```python
from build123d import *

# Parameters (mm, degrees)
SKETCH1_R           = 6.3627
BOSS_EXTRUDE1_DEPTH = 3.048
FILLET1_R           = 1.27


with BuildPart() as part:
    # Sketch1 → Boss-Extrude1 (new body, symmetric)
    with BuildSketch(Plane.XY):
        with BuildLine():
            ThreePointArc((-44.45, -20.32), (-30.440021806, -27.674009584), (-19.05, -38.657103373))
            Line((-19.05, -38.657103373), (-19.05, 38.657103373))
            ThreePointArc((-19.05, 38.657103373), (-30.440021806, 27.674009584), (-44.45, 20.32))
            ThreePointArc((-44.45, 20.32), (-30.081590206, 14.368409794), (-24.13, 0))
            ThreePointArc((-24.13, 0), (-30.081590206, -14.368409794), (-44.45, -20.32))
        make_face()
        with BuildLine():
            ThreePointArc((-19.05, -38.657103373), (-17.322621511, -40.998313496), (-15.719319348, -43.426177466))
            ThreePointArc((-15.719319348, -43.426177466), (1.415517775, -24.650338319), (7.62, 0))
            ThreePointArc((7.62, 0), (1.415517775, 24.650338319), (-15.719319348, 43.426177466))
            ThreePointArc((-15.719319348, 43.426177466), (-17.322621511, 40.998313496), (-19.05, 38.657103373))
            Line((-19.05, 38.657103373), (-19.05, -38.657103373))
        make_face()
        with BuildLine():
            ThreePointArc((-15.719319348, -43.426177466), (-9.406121761, -57.631125381), (-7.246114065, -73.025))
            Line((-7.246114065, -73.025), (19.05, -73.025))
            Line((19.05, -73.025), (19.05, 73.025))
            Line((19.05, 73.025), (-7.246114065, 73.025))
            ThreePointArc((-7.246114065, 73.025), (-9.406121761, 57.631125381), (-15.719319348, 43.426177466))
            ThreePointArc((-15.719319348, 43.426177466), (1.415517775, 24.650338319), (7.62, 0))
            ThreePointArc((7.62, 0), (1.415517775, -24.650338319), (-15.719319348, -43.426177466))
        make_face()
        with Locations((6.35, -60.325)):
            Circle(SKETCH1_R, mode=Mode.SUBTRACT)
        with Locations((6.35, 60.325)):
            Circle(SKETCH1_R, mode=Mode.SUBTRACT)
    extrude(amount=BOSS_EXTRUDE1_DEPTH, both=True)

    # Fillet1
    fillet1_edges = [part.edges().sort_by_distance(p)[0] for p in [
        (-44.45, -20.32, 0),
        (-44.45, 20.32, 0),
    ]]
    fillet(fillet1_edges, radius=FILLET1_R)


solid = part.part
```
Could you check a few things on this model? Use its own coordinates, in mm. Coordinates: 2 decimals unless noted, no trailing zeros. Write each loop counter-clockwise with the first axis right and the second up, starting at its lowest first coordinate (ties: lowest second). Pieces come first, ordered by that corner, then holes. Notation, with made-up numbers: (-30.75, -29.75) -> (-6.75, -29.75) arc R20 cw to (-6.75, -16.75) -> close; hole circle Ø5 at (48.25, 89.5). An arc over 180 degrees is marked (long way). Return JSON: item names as keys, results as strings.
(1) Imagine slicing it at B-B, the plane x = -33.5. Please give me the cut outline in (y, z), then the cut area to 3 significant figures.
Numbers:
{"outline": "(-25.61, -3.05) -> (-17.12, -3.05) -> (-17.12, 3.05) -> (-25.61, 3.05) -> close; (17.12, -3.05) -> (25.61, -3.05) -> (25.61, 3.05) -> (17.12, 3.05) -> close", "area": "104 mm2"}
(2) I need wall thicknesses on L1, parallel to Y at x = 6.35, z = -1.7 (3 decimals); L2, parallel to Y at x = 3, z = -0.5 (3 decimals); L3, parallel to X at y = 64, z = 0. Which ranges of each line are inside material? Lowest first, please.
Numbers:
{"L1": "y = -73.025 to -66.688, -53.962 to 53.962, 66.688 to 73.025", "L2": "y = -73.025 to -65.734, -54.916 to 54.916, 65.734 to 73.025", "L3": "x = -7.98 to 1.16, 11.54 to 19.05"}
(3) Imagine slicing it at A-A, the plane x = 6.35. Please give me the cut outline in (y, z) (3 decimals).
Numbers:
{"outline": "(-73.025, -3.048) -> (-66.688, -3.048) -> (-66.688, 3.048) -> (-73.025, 3.048) -> close; (-53.962, -3.048) -> (53.962, -3.048) -> (53.962, 3.048) -> (-53.962, 3.048) -> close; (66.688, -3.048) -> (73.025, -3.048) -> (73.025, 3.048) -> (66.688, 3.048) -> close"}
(4) I'm going to push flat-ended pins straight in: pin 1 (2 mm diameter, centred on x = -32, z = -0.5, fed in from +Y); pin 2 (1 mm diameter, centred on x = -32, z = -0.5, fed in from +Y); pin 3 (1 mm diameter, centred on x = -13.5, z = -0.5, fed in from -Y); pin 4 (7.5 mm diameter, centred on x = 6.35, y = -60.325, fed in from +Z). Where does each tip first touch, or does it pass through?
Numbers:
{"pin 1": "stops at y = 27.27", "pin 2": "stops at y = 26.93", "pin 3": "stops at y = -48.32", "pin 4": "passes through"}
(5) Imagine slicing it at C-C, the plane y = 30.5. Please give me the cut outline in (x, z).
Numbers:
{"outline": "(-26.84, -3.05) -> (19.05, -3.05) -> (19.05, 3.05) -> (-26.84, 3.05) -> close"}
(6) Imagine slicing it at D-D, the plane z = -1.75. Count the separate pieces of the cut face and the enclosed holes in it, then the cut area to 3 significant figures.
Numbers:
{"separate pieces": "1", "enclosed holes": "2", "area": "5,510 mm2"}
